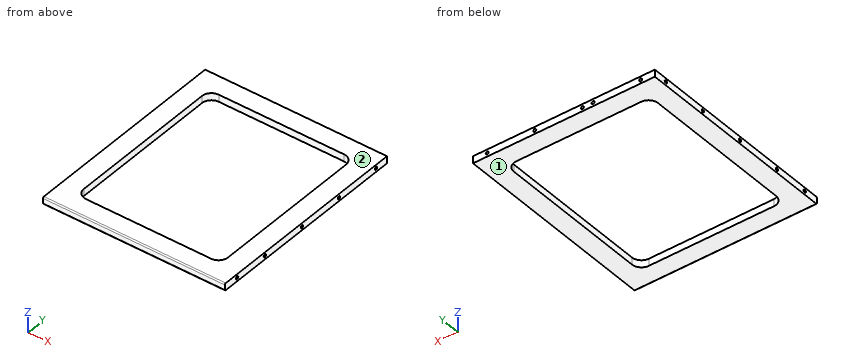
from build123d import *

# Parameters (mm, degrees)
F0_W      = 488.95
F0_H      = 560.3875
F1_DEPTH  = 19.05
F3_R      = 4
F4_DEPTH  = 26.9875
F5_SIZE   = 1.5875
F13_ANGLE = 90
F23_DEPTH = 19.051
F24_R     = 3.175


with BuildPart() as f1:
    # F0 (on Top) → F1 (new body)
    with BuildSketch(Plane.XY):
        Rectangle(F0_W, F0_H)
    extrude(amount=-F1_DEPTH)


with BuildPart() as f4:
    # F3 (on Right) → F4 (new body)
    with BuildSketch(Plane.YZ):
        with Locations((-271.8283832073, -132.3440223932)):
            Circle(F3_R)
    extrude(amount=-F4_DEPTH)

    # F5
    f5_edges = [f4.edges().sort_by_distance(p)[0] for p in [
        (-26.9875, -275.828383, -132.344022),
    ]]
    chamfer(f5_edges, length=F5_SIZE)


with BuildPart() as f6_1:
    # F6: copy of F4
    add(f4.part.moved(Location((244.475, 33.9221332073, 122.8190223932))))


with BuildPart() as f7_1:
    # F7: copy of F4
    add(f4.part.moved(Location((244.475, 129.9221332073, 122.8190223932))))


with BuildPart() as f8_1:
    # F8: copy of F4
    add(f4.part.moved(Location((244.475, 257.9221332073, 122.8190223932))))


with BuildPart() as f9_1:
    # F9: copy of F4
    add(f4.part.moved(Location((244.475, 385.9221332073, 122.8190223932))))


with BuildPart() as f10_1:
    # F10: copy of F4
    add(f4.part.moved(Location((244.475, 513.9221332073, 122.8190223932))))


with BuildPart() as f11_1:
    # F11: instance of F6_1
    add(f6_1.part.mirror(Plane.YZ))


with BuildPart() as f11_2:
    # F11: instance of F7_1
    add(f7_1.part.mirror(Plane.YZ))


with BuildPart() as f11_3:
    # F11: instance of F8_1
    add(f8_1.part.mirror(Plane.YZ))


with BuildPart() as f11_4:
    # F11: instance of F9_1
    add(f9_1.part.mirror(Plane.YZ))


with BuildPart() as f11_5:
    # F11: instance of F10_1
    add(f10_1.part.mirror(Plane.YZ))


with BuildPart() as f1_1:
    add(f1.part)

    # F12: cut F11_1, F11_2, F11_3, F11_4, F11_5, F10_1, F9_1, F8_1, F7_1, F6_1
    add(f11_1.part, mode=Mode.SUBTRACT)
    add(f11_2.part, mode=Mode.SUBTRACT)
    add(f11_3.part, mode=Mode.SUBTRACT)
    add(f11_4.part, mode=Mode.SUBTRACT)
    add(f11_5.part, mode=Mode.SUBTRACT)
    add(f10_1.part, mode=Mode.SUBTRACT)
    add(f9_1.part, mode=Mode.SUBTRACT)
    add(f8_1.part, mode=Mode.SUBTRACT)
    add(f7_1.part, mode=Mode.SUBTRACT)
    add(f6_1.part, mode=Mode.SUBTRACT)


with BuildPart() as f4_1:
    # F13: moved
    add(f4.part.rotate(Axis((244.475, -280.19375, -9.525), (0, 0, 1)), F13_ANGLE))


with BuildPart() as f16_1:
    # F16: copy of F4
    add(f4_1.part.moved(Location((-442.4846332073, 804.8625, 122.8190223932))))


with BuildPart() as f17_1:
    # F17: copy of F4
    add(f4_1.part.moved(Location((-314.4846332073, 804.8625, 122.8190223932))))


with BuildPart() as f18_1:
    # F18: copy of F4
    add(f4_1.part.moved(Location((-285.7346332073, 804.8625, 122.8190223932))))


with BuildPart() as f19_1:
    # F19: copy of F4
    add(f4_1.part.moved(Location((-157.7346332073, 804.8625, 122.8190223932))))


with BuildPart() as f4_2:
    # F20: moved
    add(f4_1.part.moved(Location((-29.7346332073, 804.8625, 122.8190223932))))


with BuildPart() as f1_2:
    add(f1_1.part)

    # F21: cut F16_1, F17_1, F18_1, F19_1, F4
    add(f16_1.part, mode=Mode.SUBTRACT)
    add(f17_1.part, mode=Mode.SUBTRACT)
    add(f18_1.part, mode=Mode.SUBTRACT)
    add(f19_1.part, mode=Mode.SUBTRACT)
    add(f4_2.part, mode=Mode.SUBTRACT)

    # F22 (on face) → F23 (cut, through all)
    with BuildSketch(Plane.XY):
        with BuildLine():
            Line((-193.675, 203.99375), (-193.675, -203.99375))
            ThreePointArc((-193.675, -203.99375), (-186.2355122421, -221.9542622421), (-168.275, -229.39375))
            Line((-168.275, -229.39375), (168.275, -229.39375))
            ThreePointArc((168.275, -229.39375), (186.2355122421, -221.9542622421), (193.675, -203.99375))
            Line((193.675, -203.99375), (193.675, 203.99375))
            ThreePointArc((193.675, 203.99375), (186.2355122421, 221.9542622421), (168.275, 229.39375))
            Line((168.275, 229.39375), (-168.275, 229.39375))
            ThreePointArc((-168.275, 229.39375), (-186.2355122421, 221.9542622421), (-193.675, 203.99375))
        make_face()
    extrude(amount=-F23_DEPTH, mode=Mode.SUBTRACT)

    # F24
    f24_edges = [f1_2.edges().sort_by_distance(p)[0] for p in [
        (0, -280.19375, 0),
        (0, -280.19375, -19.05),
    ]]
    fillet(f24_edges, radius=F24_R)


solid = f1_2.part
Geometry: final body of the model. Coordinates: model frame, mm. Face numbers are marked on the shaded views. Round coordinates to 2 decimals unless told otherwise and drop trailing zeros. Order: outer loops, then holes, each group sorted by start corner. A loop starts at its lowest first (then second) coordinate and runs counter-clockwise, first axis right, second up.
Q1. Section B-B, the plane y = 94.5. Output: boundary loops of the cut face in (x, z) (3 decimals).
Result sheet:
outline: (-244.475, -19.05) - (-193.675, -19.05) - (-193.675, 0) - (-244.475, 0) - close; (193.675, -19.05) - (244.475, -19.05) - (244.475, 0) - (193.675, 0) - close
Q2. Pin query (flat end, axial travel): pin 1 (5.5 mm diameter, centred on y = -238, z = -9.5, fed in from -X); pin 2 (4 mm diameter, centred on x = 207, z = -9, fed in from +Y); pin 3 (7 mm diameter, centred on y = -237.91, z = -9.52, fed in from +X). Return the tip coordinate at first contact, or that it passes through.
Result sheet:
pin 1: stops at x = -217.92
pin 2: stops at y = 253.61
pin 3: stops at x = 218.58
Q3. Mould query, pull axis Z, two halves, no side actions, for the marked faces 1 and 2. Classes: released by +Z, released by -Z, zero draft, split by the parting line, or undercut.
Result sheet:
face 1: released by -Z
face 2: released by +Z
Q4. Section A-A, the plane x = 140. Output: boundary loops of the cut face in (y, z) (3 decimals), and give its area (3 significant figures).
Result sheet:
outline: (-280.194, -15.875) arc R3.175 ccw to (-277.019, -19.05) - (-229.394, -19.05) - (-229.394, 0) - (-277.019, 0) arc R3.175 ccw to (-280.194, -3.175) - close; (229.394, -19.05) - (280.194, -19.05) - (280.194, 0) - (229.394, 0) - close
area: 1,930 mm2
Q5. Material intervals for probe 1 along X at (y, z) = (-122.5, -5.5) (3 decimals); probe 2 along Y at (x, z) = (127, -15.75); probe 3 along Y at (x, z) = (-51, -10), sorted ascending.
Result sheet:
probe 1: x = -244.475 to -193.675, 193.675 to 244.475
probe 2: y = -280.19 to -229.39, 229.39 to 280.19
probe 3: y = -280.19 to -229.39, 229.39 to 253.21
